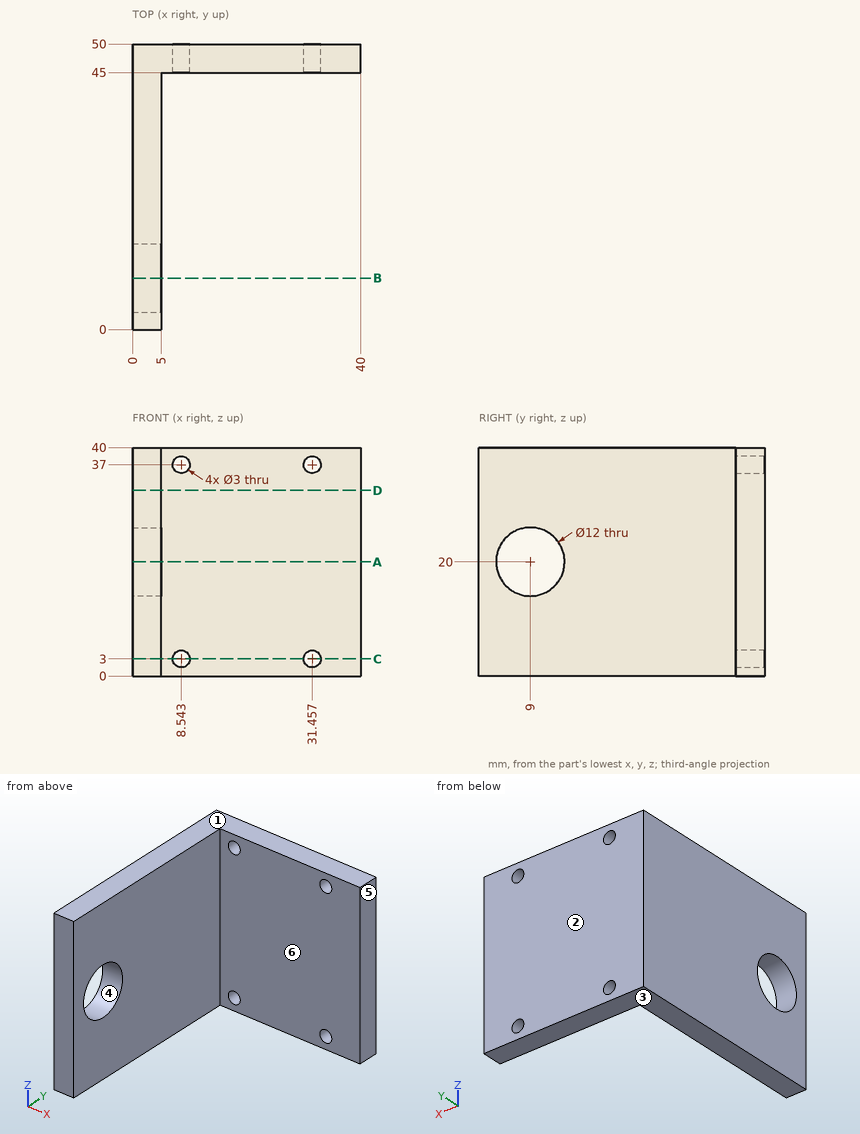
Part print with two shaded views. Sizes in mm from the minimum x, y, z corner. A direction names the side the tool comes from. Round coordinates to 2 decimals unless told otherwise and drop trailing zeros. Order: outer loops, then holes, each group sorted by start corner. A loop starts at its lowest first (then second) coordinate and runs counter-clockwise, first axis right, second up. Notation, with made-up numbers: (0, 39) - (46, 39) arc R6 ccw to (46, 48) - close; hole circle Ø3 at (18.5, 32). An arc over 180 degrees is marked (long way). Answer in a Markdown table with one row per item. Add a question column.
(1) Probe L1, parallel to X at y = 46.9, z = 37; L2, parallel to Y at x = 7.5, z = 32; L3, parallel to X at y = 31, z = 16.5. List the from-to ranges inside material, lowest first. Write a range as [from, to].
(2) Band-saw the part on D-D on z = 32.5. List the corners of the cut face in (x, y), and give its area (3 significant figures).
(3) Band-saw the part on B-B on y = 9. List the corners of the cut face in (x, z).
(4) Band-saw the part on A-A on z = 20. List the corners of the cut face in (x, y).
(5) Mould opens along Z. For the marked faces 1, 2, 3 and 4 say: +Z half, -Z half, draft (parallel to the pull), parting line (faces both ways), or undercut.
(6) 3-axis set-ups, long thin cutter, end or side, ignore diameter. For the marked faces 5 and 6: which of +Z, -Z, +X, -X, +Y, -Y reach the whole face in a straight line?
(7) Drop flat-ended pins along their axis: pin 1 Ø3.5 at (x, z) = (31.46, 37) entering from -Y; pin 2 Ø12 at (y, z) = (17.5, 17.5) entering from +X. Give the stop position or say it passes through.
(8) Band-saw the part on C-C on z = 3. List the corners of the cut face in (x, y).
Data:
| question | item | result |
|---|---|---|
| 1 | L1 | x = [0, 7.04], [10.04, 29.96], [32.96, 40] |
| 1 | L2 | y = [45, 50] |
| 1 | L3 | x = [0, 5] |
| 2 | outline | (0, 0) - (5, 0) - (5, 45) - (40, 45) - (40, 50) - (0, 50) - close |
| 2 | area | 425 mm^2 |
| 3 | outline | (0, 0) - (5, 0) - (5, 14) - (0, 14) - close; (0, 26) - (5, 26) - (5, 40) - (0, 40) - close |
| 4 | outline | (0, 0) - (5, 0) - (5, 3) - (0, 3) - close; (0, 15) - (5, 15) - (5, 45) - (40, 45) - (40, 50) - (0, 50) - close |
| 5 | face 1 | +Z half |
| 5 | face 2 | draft |
| 5 | face 3 | -Z half |
| 5 | face 4 | undercut |
| 6 | face 5 | +Z, -Z, +X, +Y, -Y |
| 6 | face 6 | +Z, -Z, +X, -Y |
| 7 | pin 1 | stops at y = 45 |
| 7 | pin 2 | stops at x = 5 |
| 8 | outline | (0, 0) - (5, 0) - (5, 45) - (7.04, 45) - (7.04, 50) - (0, 50) - close; (10.04, 45) - (29.96, 45) - (29.96, 50) - (10.04, 50) - close; (32.96, 45) - (40, 45) - (40, 50) - (32.96, 50) - close |
